Geometry check sheet. Reference: the model listing, model coordinates, mm. Coordinates: 2 decimals unless noted, no trailing zeros. Loops run counter-clockwise (first coordinate to the right, second up) from the corner with the lowest first, then second, coordinate; pieces in that order, holes last.
from build123d import *

# Parameters (mm, degrees)
SKETCH1_W               = 88.5
SKETCH1_H               = 60.5
BOSS_EXTRUDE1_DEPTH     = 3
SKETCH2_W               = 55.9
SKETCH2_H               = 3
BOSS_EXTRUDE2_DEPTH     = 5.375
SKETCH3_W               = 14
SKETCH3_H               = 14
CUT_EXTRUDE4_DEPTH      = 112.72182251
SKETCH7_W               = 20
SKETCH7_H               = 20
CUT_EXTRUDE5_DEPTH      = 1.5
SKETCH9_W               = 15
SKETCH9_H               = 3
CUT_EXTRUDE6_DEPTH      = 3
SKETCH10_W              = 14
SKETCH10_H              = 14
CUT_EXTRUDE7_DEPTH      = 10
SKETCH11_W              = 20
SKETCH11_H              = 20
CUT_EXTRUDE8_DEPTH      = 1.5
SKETCH12_W              = 15
SKETCH12_H              = 3
CUT_EXTRUDE9_DEPTH      = 40
MIRROR8_COPY_1_SKETCH_W = 14
MIRROR8_COPY_1_SKETCH_H = 14
MIRROR8_COPY_1_DEPTH    = 112.72182251
MIRROR8_COPY_2_SKETCH_W = 20
MIRROR8_COPY_2_SKETCH_H = 20
MIRROR8_COPY_2_DEPTH    = 1.5
SKETCH13_W              = 5.375
SKETCH13_H              = 2.3
BOSS_EXTRUDE3_DEPTH     = 3
SKETCH15_W              = 15
SKETCH15_H              = 5
CUT_EXTRUDE11_DEPTH     = 112.72182251


with BuildPart() as part:
    # Sketch1 → Boss-Extrude1 (new body)
    with BuildSketch(Plane(origin=(0, 0, 0), x_dir=(1, 0, 0), z_dir=(0, 1, 0))):
        with Locations((44.25, 30.25)):
            Rectangle(SKETCH1_W, SKETCH1_H)
    extrude(amount=BOSS_EXTRUDE1_DEPTH)

    # Sketch2 → Boss-Extrude2 (add)
    with BuildSketch(Plane(origin=(88.5, 0, 0), x_dir=(0, 0, -1), z_dir=(1, 0, 0))):
        with Locations((30.25, 1.5)):
            Rectangle(SKETCH2_W, SKETCH2_H)
    boss_extrude2 = extrude(amount=BOSS_EXTRUDE2_DEPTH)

    # Mirror2: Boss-Extrude2 across plane
    add(boss_extrude2.mirror(Plane(origin=(44.25, 0, 0), x_dir=(0, 0, 1), z_dir=(1, 0, 0))))

    # Sketch3 → Cut-Extrude4 (cut, through all)
    with BuildSketch(Plane.XZ):
        with Locations((20.25, -44.25)):
            Rectangle(SKETCH3_W, SKETCH3_H)
    cut_extrude4 = extrude(amount=-CUT_EXTRUDE4_DEPTH, mode=Mode.SUBTRACT)

    # Sketch7 → Cut-Extrude5 (cut)
    with BuildSketch(Plane.XZ):
        with Locations((20.25, -44.25)):
            Rectangle(SKETCH7_W, SKETCH7_H)
    cut_extrude5 = extrude(amount=-CUT_EXTRUDE5_DEPTH, mode=Mode.SUBTRACT)

    # Mirror4: Cut-Extrude4, Cut-Extrude5 across plane
    add(cut_extrude4.mirror(Plane(origin=(44.25, 0, 0), x_dir=(0, 0, 1), z_dir=(1, 0, 0))), mode=Mode.SUBTRACT)
    add(cut_extrude5.mirror(Plane(origin=(44.25, 0, 0), x_dir=(0, 0, 1), z_dir=(1, 0, 0))), mode=Mode.SUBTRACT)

    # Sketch9 → Cut-Extrude6 (cut)
    with BuildSketch(Plane(origin=(0, 0, -60.5), x_dir=(-1, 0, 0), z_dir=(0, 0, -1))):
        with Locations((-20.25, 1.5)):
            Rectangle(SKETCH9_W, SKETCH9_H)
    cut_extrude6 = extrude(amount=-CUT_EXTRUDE6_DEPTH, mode=Mode.SUBTRACT)

    # Mirror6: Cut-Extrude6 across plane
    add(cut_extrude6.mirror(Plane(origin=(44.25, 0, 0), x_dir=(0, 0, 1), z_dir=(1, 0, 0))), mode=Mode.SUBTRACT)

    # Sketch10 → Cut-Extrude7 (cut)
    with BuildSketch(Plane(origin=(0, 3, 0), x_dir=(1, 0, 0), z_dir=(0, 1, 0))):
        with Locations((44.25, 44.25)):
            Rectangle(SKETCH10_W, SKETCH10_H)
    cut_extrude7 = extrude(amount=-CUT_EXTRUDE7_DEPTH, mode=Mode.SUBTRACT)

    # Sketch11 → Cut-Extrude8 (cut)
    with BuildSketch(Plane.XZ):
        with Locations((44.25, -44.25)):
            Rectangle(SKETCH11_W, SKETCH11_H)
    cut_extrude8 = extrude(amount=-CUT_EXTRUDE8_DEPTH, mode=Mode.SUBTRACT)

    # Sketch12 → Cut-Extrude9 (cut)
    with BuildSketch(Plane.XZ):
        with Locations((44.25, -59)):
            Rectangle(SKETCH12_W, SKETCH12_H)
    extrude(amount=-CUT_EXTRUDE9_DEPTH, mode=Mode.SUBTRACT)

    # Mirror8: Cut-Extrude4, Cut-Extrude5, Cut-Extrude7, Cut-Extrude8 across plane
    add(cut_extrude4.mirror(Plane.XY.offset(-30)), mode=Mode.SUBTRACT)
    add(cut_extrude5.mirror(Plane.XY.offset(-30)), mode=Mode.SUBTRACT)
    add(cut_extrude7.mirror(Plane.XY.offset(-30)), mode=Mode.SUBTRACT)
    add(cut_extrude8.mirror(Plane.XY.offset(-30)), mode=Mode.SUBTRACT)

    # Mirror8 copy 1 sketch → Mirror8 copy 1 (cut, through all)
    with BuildSketch(Plane(origin=(88.5, 0, -60), x_dir=(-1, 0, 0), z_dir=(0, -1, 0))):
        with Locations((20.25, -44.25)):
            Rectangle(MIRROR8_COPY_1_SKETCH_W, MIRROR8_COPY_1_SKETCH_H)
    extrude(amount=-MIRROR8_COPY_1_DEPTH, mode=Mode.SUBTRACT)

    # Mirror8 copy 2 sketch → Mirror8 copy 2 (cut)
    with BuildSketch(Plane(origin=(88.5, 0, -60), x_dir=(-1, 0, 0), z_dir=(0, -1, 0))):
        with Locations((20.25, -44.25)):
            Rectangle(MIRROR8_COPY_2_SKETCH_W, MIRROR8_COPY_2_SKETCH_H)
    extrude(amount=-MIRROR8_COPY_2_DEPTH, mode=Mode.SUBTRACT)

    # Sketch13 → Boss-Extrude3 (add)
    with BuildSketch(Plane(origin=(0, 3, 0), x_dir=(1, 0, 0), z_dir=(0, 1, 0))):
        with Locations((-2.6875, 59.35)):
            Rectangle(SKETCH13_W, SKETCH13_H)
        with Locations((-2.6875, 1.15)):
            Rectangle(SKETCH13_W, SKETCH13_H)
        with Locations((91.1875, 1.15)):
            Rectangle(SKETCH13_W, SKETCH13_H)
        with Locations((91.1875, 59.35)):
            Rectangle(SKETCH13_W, SKETCH13_H)
    extrude(amount=-BOSS_EXTRUDE3_DEPTH)

    # Sketch15 → Cut-Extrude11 (cut, through all)
    with BuildSketch(Plane.XZ):
        with Locations((20.25, -29.75)):
            Rectangle(SKETCH15_W, SKETCH15_H)
        with Locations((44.25, -29.75)):
            Rectangle(SKETCH15_W, SKETCH15_H)
        with Locations((68.25, -29.75)):
            Rectangle(SKETCH15_W, SKETCH15_H)
    extrude(amount=-CUT_EXTRUDE11_DEPTH, mode=Mode.SUBTRACT)


solid = part.part
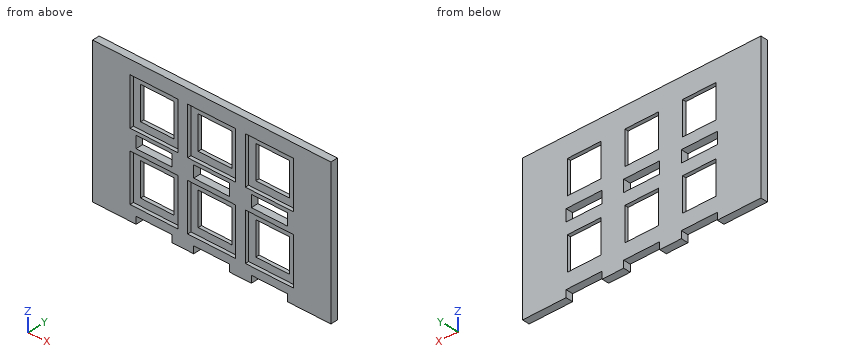
(1) Sectioned sample at A-A on z = -30. Record the cut outline in (x, y) (3 decimals), and give its area (3 significant figures).
Findings:
outline: (-5.375, 0) - (12.75, 0) - (12.75, 3) - (-5.375, 3) - close; (27.75, 0) - (36.75, 0) - (36.75, 3) - (27.75, 3) - close; (51.75, 0) - (60.75, 0) - (60.75, 3) - (51.75, 3) - close; (75.75, 0) - (93.875, 0) - (93.875, 3) - (75.75, 3) - close
area: 163 mm2
(2) Scan lines: L1, parallel to X at y = 2.05, z = -48 (3 decimals); L2, parallel to Z at x = 61.5, y = 0.55; L3, parallel to X at y = 0.5, z = -10 (3 decimals). Record each from-to range of solid material in increasing order.
Findings:
L1: x = -5.375 to 13.25, 27.25 to 37.25, 51.25 to 61.25, 75.25 to 93.875
L2: z = -57.5 to -54.25, -34.25 to -32.25, -27.25 to -25.75, -5.75 to 0
L3: x = -5.375 to 10.25, 30.25 to 34.25, 54.25 to 58.25, 78.25 to 93.875
(3) Sectioned sample at C-C on x = 11.5. Record the cut outline in (y, z).
Findings:
outline: (0, -60.5) - (3, -60.5) - (3, 0) - (0, 0) - (0, -5.75) - (1.5, -5.75) - (1.5, -25.75) - (0, -25.75) - (0, -34.25) - (1.5, -34.25) - (1.5, -54.25) - (0, -54.25) - close
(4) Gauge pin test, flat ends, axial feed: pin 1 Ø1.6 at (x, y) = (45, 1) entering from +Z; pin 2 Ø1.6 at (x, y) = (18.5, 2) entering from -Z. Record the tip position at first contact, or that the pin passes through.
Findings:
pin 1: stops at z = 0
pin 2: stops at z = -57.5
(5) Sectioned sample at B-B on x = 24.5. Record the cut outline in (y, z).
Findings:
outline: (0, -57.5) - (3, -57.5) - (3, -51.25) - (1.5, -51.25) - (1.5, -54.25) - (0, -54.25) - close; (0, -34.25) - (1.5, -34.25) - (1.5, -37.25) - (3, -37.25) - (3, -32.25) - (0, -32.25) - close; (0, -27.25) - (3, -27.25) - (3, -22.75) - (1.5, -22.75) - (1.5, -25.75) - (0, -25.75) - close; (0, -5.75) - (1.5, -5.75) - (1.5, -8.75) - (3, -8.75) - (3, 0) - (0, 0) - close
(6) Sectioned sample at D-D on z = -10. Record the cut outline in (x, y) (3 decimals), and give its area (3 significant figures).
Findings:
outline: (-5.375, 0) - (10.25, 0) - (10.25, 1.5) - (13.25, 1.5) - (13.25, 3) - (-5.375, 3) - close; (27.25, 1.5) - (30.25, 1.5) - (30.25, 0) - (34.25, 0) - (34.25, 1.5) - (37.25, 1.5) - (37.25, 3) - (27.25, 3) - close; (51.25, 1.5) - (54.25, 1.5) - (54.25, 0) - (58.25, 0) - (58.25, 1.5) - (61.25, 1.5) - (61.25, 3) - (51.25, 3) - close; (75.25, 1.5) - (78.25, 1.5) - (78.25, 0) - (93.875, 0) - (93.875, 3) - (75.25, 3) - close
area: 145 mm2
